```python
from build123d import *

# Parameters (mm, degrees)
SKETCH1_W           = 6
SKETCH1_H           = 6
BOSS_EXTRUDE1_DEPTH = 5
CUT_EXTRUDE12_DEPTH = 3.5
CUT_EXTRUDE13_DEPTH = 3.5
CUT_EXTRUDE14_DEPTH = 3.5


with BuildPart() as part:
    # Sketch1 → Boss-Extrude1 (new body)
    with BuildSketch(Plane(origin=(0, 0, 0), x_dir=(1, 0, 0), z_dir=(0, 1, 0))):
        Rectangle(SKETCH1_W, SKETCH1_H)
    extrude(amount=BOSS_EXTRUDE1_DEPTH)

    # Sketch13 → Cut-Extrude12 (cut)
    with BuildSketch(Plane(origin=(0, 0, -3), x_dir=(-1, 0, 0), z_dir=(0, 0, -1))):
        with BuildLine():
            ThreePointArc((-3, 5), (0.780941195, 3.437129434), (3, 0))
            Line((3, 0), (3, 5))
            Line((3, 5), (-3, 5))
        make_face()
    extrude(amount=-CUT_EXTRUDE12_DEPTH, mode=Mode.SUBTRACT)

    # Sketch14 → Cut-Extrude13 (cut)
    with BuildSketch(Plane(origin=(0, 0, 0.5), x_dir=(-1, 0, 0), z_dir=(0, 0, -1))):
        with BuildLine():
            ThreePointArc((-3, 5), (-1.441597312, 4.675208063), (0, 4))
            Line((0, 4), (0, 5))
            Line((0, 5), (-3, 5))
        make_face()
    extrude(amount=-CUT_EXTRUDE13_DEPTH, mode=Mode.SUBTRACT)

    # Sketch15 → Cut-Extrude14 (cut)
    with BuildSketch(Plane.XY.offset(3)):
        Polygon((-3, 4), (0, 5), (-3, 5), align=None)
        Polygon((0, 1), (-3, 3), (-3, 0), (0, 0), align=None)
    extrude(amount=-CUT_EXTRUDE14_DEPTH, mode=Mode.SUBTRACT)


solid = part.part
```
The listing builds one solid part. Answer for the finished solid, in the listing's coordinates (mm). A direction names the side the tool comes from. Give positions to 0.01 mm unless a question says otherwise; leave off trailing zeros. Write each loop counter-clockwise with the first axis right and the second up, starting at its lowest first coordinate (ties: lowest second). Pieces come first, ordered by that corner, then holes. Notation, with made-up numbers: (77.25, -39.5) -> (98.25, -39.5) arc R23 ccw to (98.25, -1.5) -> close; hole circle Ø6 at (-22, 63.25). An arc over 180 degrees is marked (long way). Write item = value, one per line. Start each with the question number.
1) Straight lines are drawn through the part: line 1 along X through (y, z) = (0.2, 1.25); line 2 along Z through (x, y) = (-0.75, 4.25); line 3 along X through (y, z) = (4.25, -1.95). For each, find the intervals that lie inside material, in ascending order.
2) The part is cut by section C-C, the plane x = -2. Determine the outline of the cut face in (y, z), and give its area (3 significant figures).
3) The part is cut by section D-D, the plane x = -1. Determine the outline of the cut face in (y, z), and give its area (3 significant figures).
4) The part is cut by section A-A, the plane y = 4.55. Determine the outline of the cut face in (x, z).
5) Each of these flat-tipped pins is pushed along its axis until it touches: pin 1 (0.8 mm diameter, centred on x = -1.5, y = 4, fed in from -Z); pin 2 (0.7 mm diameter, centred on x = -1.5, y = 1.5, fed in from +Z); pin 3 (0.5 mm diameter, centred on y = 0.5, z = 1.5, fed in from -X). Where does it stop, or does it pass through?
6) Determine the mould class of faces 4 (the face through (1, 0, -1)), 5 (the face through (-1.5, 2, 1.3)), 6 (the face through (0, 4.5, 1.7)) for opening direction X: +X half, -X half, draft (parallel to the pull), parting line (faces both ways), or undercut.
7) Which of the six approach directions +Z, -Z, +X, -X, +Y, -Y give full straight-line access (tool end or side, diameter ignored) to faces 1 (the face through (-1, 4, 0.5)), 2 (the face through (3, 2, 0)), 3 (the face through (-2, 1, -0.5))?
8) The part is cut by section B-B, the plane z = 1.7. Determine the outline of the cut face in (x, y).
Solutions:
q1.line_1 = 0 to 3
q1.line_2 = 0.5 to 3
q1.line_3 = 0.44 to 3
q2.outline = (0, -3) -> (2.11, -3) -> (2.11, -0.5) -> (0, -0.5) -> close; (2.33, 0.5) -> (4.33, 0.5) -> (4.33, 3) -> (2.33, 3) -> close
q2.area = 10.3 mm²
q3.outline = (0, -3) -> (3.25, -3) -> (3.25, 0.5) -> (4.67, 0.5) -> (4.67, 3) -> (1.67, 3) -> (1.67, -0.5) -> (0, -0.5) -> close
q3.area = 17.2 mm²
q4.outline = (-1.35, 0.5) -> (0, 0.5) -> (0, 3) -> (-1.35, 3) -> close; (1.1, -3) -> (3, -3) -> (3, 3) -> (1.1, 3) -> close
q5.pin_1 = 0.5
q5.pin_2 = -0.5
q5.pin_3 = 0
q6.face_4 = draft
q6.face_5 = -X half
q6.face_6 = undercut
q7.face_1 = -Z, -X, +Y
q7.face_2 = +Z, -Z, +X, +Y, -Y
q7.face_3 = +Z, -X, -Y
q8.outline = (-3, 3) -> (0, 1) -> (0, 0) -> (3, 0) -> (3, 5) arc R6.86 ccw to (0, 4) -> (0, 5) -> (-3, 4) -> close
